Input: part model. Units: mm. Frame: model coordinates. A direction names the side the tool comes from. Round coordinates to 2 decimals unless told otherwise and drop trailing zeros. Loops run counter-clockwise (first coordinate to the right, second up) from the corner with the lowest first, then second, coordinate; pieces in that order, holes last. Notation, with made-up numbers: M 79.5,1.5 L 132.5,1.5 A23 ccw 132.5,32.5 Z; hole C 2,53.25 d2. An arc over 180 degrees is marked long. Put each result on its own line as item: value. Start each with the question number.
1) Pin query (flat end, axial travel): pin 1 (2 mm diameter, centred on x = 35, z = -42.5, fed in from +Y); pin 2 (8 mm diameter, centred on x = 25, z = -38, fed in from +Y); pin 3 (2.5 mm diameter, centred on x = 11.5, z = -5, fed in from +Y); pin 4 (3 mm diameter, centred on y = 8, z = -30.5, fed in from +X). Return the tip coordinate at first contact, or that it passes through.
2) Section D-D on x = 50. Output: boundary loops of the cut face in (y, z).
3) Line query: probe 1 along X at (y, z) = (6.7, -5); probe 2 along Z at (x, y) = (34, 3.8); probe 3 along Y at (x, z) = (44.5, -3). Output: solid intervals per line, ascending.
4) Section C-C on y = 3. Output: boundary loops of the cut face in (x, z), plus the area to 3 significant figures.
5) Draft query along Z for faces 1 (the face through (35.4, 2, -8.9)), 2 (the face through (52, 10, -6.3)), 3 (the face through (13.586, 7.219, -45.208)), 4 (the face through (0.57, 2.54, -0.6)). Return one class per face: +Z half, -Z half, draft (parallel to the pull), parting line (faces both ways), or undercut.
6) Reachability of faces 5 (the face through (35.03, 1.01, -43.85)), 6 (the face through (13.586, 7.219, -5.208)) from +Z, -Z, +X, -X, +Y, -Y: full face, straight path, thin tool, end or side. Return the list, or none.
7) Section A-A on y = 7.75. Output: boundary loops of the cut face in (x, z), plus the area to 3 significant figures.
8) Section B-B on x = 34. Output: boundary loops of the cut face in (y, z) (3 decimals).
from build123d import *

# Parameters (mm, degrees)
SKETCH1_W                     = 54
SKETCH1_H                     = 50
BOSS_EXTRUDE1_DEPTH           = 5
SKETCH2_R                     = 3
SKETCH2_R_2                   = 1.6
BOSS_EXTRUDE2_DEPTH           = 5
CBORE_FOR_M3_SHCS1_AT_2_COUNT = 2
CBORE_FOR_M3_SHCS1_AT_2_PITCH = 35
CHAMFER1_SIZE                 = 0.5
FILLET1_R                     = 2


with BuildPart() as part:
    # Sketch1 → Boss-Extrude1 (new body)
    with BuildSketch(Plane(origin=(0, 0, 0), x_dir=(1, 0, 0), z_dir=(0, 1, 0))):
        with Locations((27, 25)):
            Rectangle(SKETCH1_W, SKETCH1_H)
    extrude(amount=BOSS_EXTRUDE1_DEPTH)

    # Sketch2 → Boss-Extrude2 (add)
    # profile 1 of 4: a face of its own
    with BuildSketch(Plane(origin=(0, 5, 0), x_dir=(1, 0, 0), z_dir=(0, 1, 0))):
        with Locations(Location((50, 5, 0), (0, 0, 90))):
            Circle(SKETCH2_R)
        with Locations(Location((50, 5, 0), (0, 0, 270))):
            Circle(SKETCH2_R_2, mode=Mode.SUBTRACT)
    # profile 2 of 4: a face of its own
    with BuildSketch(Plane(origin=(0, 5, 0), x_dir=(1, 0, 0), z_dir=(0, 1, 0))):
        with Locations(Location((50, 45, 0), (0, 0, 90))):
            Circle(SKETCH2_R)
        with Locations(Location((50, 45, 0), (0, 0, 270))):
            Circle(SKETCH2_R_2, mode=Mode.SUBTRACT)
    # profile 3 of 4: a face of its own
    with BuildSketch(Plane(origin=(0, 5, 0), x_dir=(1, 0, 0), z_dir=(0, 1, 0))):
        with Locations(Location((12, 45, 0), (0, 0, 90))):
            Circle(SKETCH2_R)
        with Locations(Location((12, 45, 0), (0, 0, 270))):
            Circle(SKETCH2_R_2, mode=Mode.SUBTRACT)
    # profile 4 of 4: a face of its own
    with BuildSketch(Plane(origin=(0, 5, 0), x_dir=(1, 0, 0), z_dir=(0, 1, 0))):
        with Locations(Location((12, 5, 0), (0, 0, 90))):
            Circle(SKETCH2_R)
        with Locations(Location((12, 5, 0), (0, 0, 270))):
            Circle(SKETCH2_R_2, mode=Mode.SUBTRACT)
    extrude(amount=BOSS_EXTRUDE2_DEPTH)

    # Sketch4 → CBORE for M3 SHCS1 (revolve, cut)
    with BuildSketch(Plane(origin=(34, 5, -42.5), x_dir=(0, 0, 1), z_dir=(1, 0, 0))):
        Polygon((0, 0), (0, 5), (1.7, 5), (1.7, 3), (3.25, 3), (3.25, 0.025), (3.275, 0), align=None)
    cbore_for_m3_shcs1 = revolve(axis=Axis((34, 11.35, -42.5), (0, -1, 0)), mode=Mode.SUBTRACT)

    # CBORE for M3 SHCS1 at 2: CBORE for M3 SHCS1 ×2
    with Locations(*[(0, 0, i * CBORE_FOR_M3_SHCS1_AT_2_PITCH) for i in range(1, CBORE_FOR_M3_SHCS1_AT_2_COUNT)]):
        add(cbore_for_m3_shcs1, mode=Mode.SUBTRACT)

    # Chamfer1
    chamfer1_edges = [part.edges().sort_by_distance(p)[0] for p in [
        (12, 10, -6.6),
        (12, 10, -46.6),
        (50, 10, -46.6),
        (50, 10, -6.6),
    ]]
    chamfer(chamfer1_edges, length=CHAMFER1_SIZE)

    # Fillet1
    fillet1_edges = [part.edges().sort_by_distance(p)[0] for p in [
        (0, 2.5, -50),
        (54, 2.5, -50),
        (54, 2.5, 0),
        (0, 2.5, 0),
    ]]
    fillet(fillet1_edges, radius=FILLET1_R)


solid = part.part
Geometry results:
1. pin 1: stops at y = 2
1. pin 2: stops at y = 5
1. pin 3: stops at y = 9.65
1. pin 4: passes through
2. outline: M 0,-50 L 5,-50 L 5,-48 L 10,-48 L 10,-47.1 L 9.5,-46.6 L 5,-46.6 L 5,-43.4 L 9.5,-43.4 L 10,-42.9 L 10,-42 L 5,-42 L 5,-8 L 10,-8 L 10,-7.1 L 9.5,-6.6 L 5,-6.6 L 5,-3.4 L 9.5,-3.4 L 10,-2.9 L 10,-2 L 5,-2 L 5,0 L 0,0 Z
3. probe 1: x = 9 to 10.4, 13.6 to 15, 47 to 48.4, 51.6 to 53
3. probe 2: z = -50 to -45.75, -39.25 to -10.75, -4.25 to 0
3. probe 3: y = 0 to 5
4. outline: M 0,-48 A2 ccw 2,-50 L 52,-50 A2 ccw 54,-48 L 54,-2 A2 ccw 52,0 L 2,0 A2 ccw 0,-2 Z; hole C 34,-42.5 d6.5; hole C 34,-7.5 d6.5
4. area: 2,630 mm²
5. face 1: undercut
5. face 2: draft
5. face 3: undercut
5. face 4: +Z half
6. face 5: +Y, -Y
6. face 6: +Y
7. outline: C 12,-45 d6; C 12,-5 d6; C 50,-45 d6; C 50,-5 d6; hole C 12,-45 d3.2; hole C 12,-5 d3.2; hole C 50,-45 d3.2; hole C 50,-5 d3.2
7. area: 80.9 mm²
8. outline: M 0,-50 L 5,-50 L 5,-45.775 L 4.975,-45.75 L 2,-45.75 L 2,-44.2 L 0,-44.2 Z; M 0,-40.8 L 2,-40.8 L 2,-39.25 L 4.975,-39.25 L 5,-39.225 L 5,-10.775 L 4.975,-10.75 L 2,-10.75 L 2,-9.2 L 0,-9.2 Z; M 0,-5.8 L 2,-5.8 L 2,-4.25 L 4.975,-4.25 L 5,-4.225 L 5,0 L 0,0 Z
